Build history of the part. All positions in model axes, mm. Face numbers are marked on the shaded views. A direction names the side the tool comes from. Give positions to 0.01 mm unless a question says otherwise; leave off trailing zeros. Order: outer loops, then holes, each group sorted by start corner. A loop starts at its lowest first (then second) coordinate and runs counter-clockwise, first axis right, second up. Notation, with made-up numbers: (70.25, 63) - (92.25, 63) arc R14 cw to (92.25, 81) - close; hole circle Ø7 at (9.25, 57.5). An arc over 180 degrees is marked (long way). Use a Markdown table: item, result.
from build123d import *

# Parameters (mm, degrees)
SKETCH1_R           = 7.5
BOSS_EXTRUDE1_DEPTH = 25
SKETCH2_R           = 5.1
CUT_EXTRUDE1_DEPTH  = 7
SKETCH3_R           = 5.1
CUT_EXTRUDE2_DEPTH  = 7
SKETCH4_R           = 4
CUT_EXTRUDE3_DEPTH  = 19


with BuildPart() as part:
    # Sketch1 → Boss-Extrude1 (new body)
    with BuildSketch(Plane(origin=(0, 0, 0), x_dir=(1, 0, 0), z_dir=(0, 1, 0))):
        Circle(SKETCH1_R)
    extrude(amount=BOSS_EXTRUDE1_DEPTH)

    # Sketch2 → Cut-Extrude1 (cut)
    with BuildSketch(Plane.XZ):
        Circle(SKETCH2_R)
    extrude(amount=-CUT_EXTRUDE1_DEPTH, mode=Mode.SUBTRACT)

    # Sketch3 → Cut-Extrude2 (cut)
    with BuildSketch(Plane(origin=(0, 25, 0), x_dir=(1, 0, 0), z_dir=(0, 1, 0))):
        Circle(SKETCH3_R)
    extrude(amount=-CUT_EXTRUDE2_DEPTH, mode=Mode.SUBTRACT)

    # Sketch4 → Cut-Extrude3 (cut, through all)
    with BuildSketch(Plane(origin=(0, 18, 0), x_dir=(1, 0, 0), z_dir=(0, 1, 0))):
        Circle(SKETCH4_R)
    extrude(amount=-CUT_EXTRUDE3_DEPTH, mode=Mode.SUBTRACT)


solid = part.part
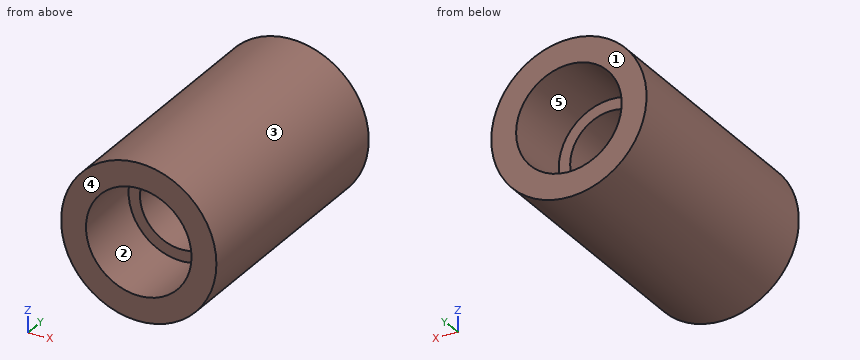
1) Slice it at A-A (x = 0). Write the cut outline in (y, z), and give its area (3 significant figures).
Computed:
| item | result |
|---|---|
| outline | (0, -7.5) - (25, -7.5) - (25, -5.1) - (18, -5.1) - (18, -4) - (7, -4) - (7, -5.1) - (0, -5.1) - close; (0, 5.1) - (7, 5.1) - (7, 4) - (18, 4) - (18, 5.1) - (25, 5.1) - (25, 7.5) - (0, 7.5) - close |
| area | 144 mm² |
2) Tool access for the marked faces 4 and 5: list every direction of +Z, -Z, +X, -X, +Y, -Y with a clear straight run to the whole face (end or side of a thin tool).
Computed:
| item | result |
|---|---|
| face 4 | +Z, -Z, +X, -X, -Y |
| face 5 | +Y |
3) Slice it at D-D (y = 19). Write the cut outline in (x, z), and give its area (3 significant figures).
Computed:
| item | result |
|---|---|
| outline | circle Ø15 at (0, 0); hole circle Ø10.2 at (0, 0) |
| area | 95.0 mm² |
4) Wall check: line 1 (Z direction, x = 0, y = 4.5); line 2 (Z direction, x = 0, y = 13.5); line 3 (X direction, y = 24, z = 0.25). Give the ranges that are in metal, low to high. Write a range as from..to.
Computed:
| item | result |
|---|---|
| line 1 | z = -7.5..-5.1, 5.1..7.5 |
| line 2 | z = -7.5..-4, 4..7.5 |
| line 3 | x = -7.5..-5.09, 5.09..7.5 |
5) Pin check, flat tips, straight feed: P1, Ø5, axis at x = -4.5, y = 11, coming from the +Z side; P2, Ø3, axis at x = 0, z = -2, coming from the -Y side; P3, Ø9, axis at x = 0, z = 0, coming from the -Y side; P4, Ø1, axis at x = 1.5, y = 17.5, coming from the +Z side. Stop position of each tip, or through.
Computed:
| item | result |
|---|---|
| P1 | stops at z = 7.23 |
| P2 | passes through |
| P3 | stops at y = 7 |
| P4 | stops at z = 7.43 |
6) Slice it at C-C (z = -4.5). Write the cut outline in (x, y), and give its area (3 significant figures).
Computed:
| item | result |
|---|---|
| outline | (-6, 0) - (-2.4, 0) - (-2.4, 7) - (2.4, 7) - (2.4, 0) - (6, 0) - (6, 25) - (2.4, 25) - (2.4, 18) - (-2.4, 18) - (-2.4, 25) - (-6, 25) - close |
| area | 233 mm² |
7) Slice it at B-B (z = 0). Write the cut outline in (x, y).
Computed:
| item | result |
|---|---|
| outline | (-7.5, 0) - (-5.1, 0) - (-5.1, 7) - (-4, 7) - (-4, 18) - (-5.1, 18) - (-5.1, 25) - (-7.5, 25) - close; (4, 7) - (5.1, 7) - (5.1, 0) - (7.5, 0) - (7.5, 25) - (5.1, 25) - (5.1, 18) - (4, 18) - close |
8) Two-plate mould, pull along Z, no slides. Class the marked faces 1, 2 and 3: +Z half, -Z half, draft (parallel to the pull), parting line (faces both ways), or undercut.
Computed:
| item | result |
|---|---|
| face 1 | draft |
| face 2 | undercut |
| face 3 | parting line |
